Design review of the part built by this model. Coordinates are the model's own, in mm. A direction names the side the tool comes from. Coordinates: 2 decimals unless noted, no trailing zeros. Loops run counter-clockwise (first coordinate to the right, second up) from the corner with the lowest first, then second, coordinate; pieces in that order, holes last.
Q1. Add section C-C on z = -29.5. Give the boundary of the cut face in (x, y).
Q2. Wall thickness on probe 1 along X at (y, z) = (1.5, -139.7); probe 2 along X at (y, z) = (4.5, -114.3): over which ranges is each line inside the solid? List them lowest first.
Q3. For P1, Ø2.5, axis at x = -144, y = 5, coming from the -Z side; P2, Ø2, axis at y = 1, z = -86.5, coming from the -X side; P3, Ø3, axis at y = 4.5, z = -162.5, coming from the -X side; P4, Ø2.5, axis at y = 4.5, z = -20.5, coming from the +X side, all flat-tipped, find the tip position at first contact; note any pin that passes through.
Q4. Add section A-A on x = -139.7. Give the boundary of the cut face in (y, z), and give its area (3 significant figures).
Q5. Machinability: for faces 1 (the face through (-25.4, 4, -126)), 2 (the face through (-21, 4, -160)), 3 (the face through (-3, 4, -80)), which of the approach directions +Z, -Z, +X, -X, +Y, -Y give a long, thin tool a straight path to every point of the face, cutting with its end or side? Answer none if there is none.
Q6. Add section D-D on x = -29. Give the boundary of the cut face in (y, z).
Q7. Draft analysis for pull direction Z (two halves, no side actions). For faces 4 (the face through (0, 4, -50)), 5 (the face through (-24.285, 4.024, -105.16)), 6 (the face through (-1.804, 4.024, -1.711)), state which applies: released by +Z, released by -Z, zero draft, split by the parting line, or undercut.
Q8. Add section B-B on y = 2. Give the number of separate pieces and of enclosed holes in the cut face, and give its area (3 significant figures).
Autodesk Inventor part; units mm, degrees
ref_plane "YZ Plane" through (0, 0, 0) normal (1, 0, 0) x (0, 1, 0)
ref_plane "XZ Plane" through (0, 0, 0) normal (0, 1, 0) x (-1, 0, 0)
ref_plane "XY Plane" through (0, 0, 0) normal (0, 0, 1) x (1, 0, 0)
sketch "Sketch1" plane through (0, 0, 0) normal (0, 1, 0) x (-1, 0, 0)
  line L0 (169.8625, 0) -> (0, 0)
  line L1 (0, 0) -> (0, -169.8625)
  line L2 (0, -169.8625) -> (25.4, -169.8625)
  line L3 (25.4, -169.8625) -> (25.4, -103.8713)
  line L4 (103.8713, -25.4) -> (169.8625, -25.4)
  line L5 (169.8625, -25.4) -> (169.8625, 0)
  arc A0 (103.8713, -25.4) -> (25.4, -103.8713) centre (66.675, -66.675) ccw
  line L6 (0, 0) -> (66.675, -66.675) construction
  line L7 (0, -20) -> (6.35, -20)
  line L8 (6.35, -20) -> (6.35, -40)
  line L9 (6.35, -40) -> (0, -40)
  line L10 (0, -40) -> (0, -20)
  line L11 (6.35, -60) -> (6.35, -80)
  line L12 (0, -60) -> (6.35, -60)
  line L13 (6.35, -80) -> (0, -80)
  line L14 (6.35, -100) -> (6.35, -120)
  line L15 (0, -100) -> (6.35, -100)
  line L16 (6.35, -120) -> (0, -120)
  line L17 (6.35, -140) -> (6.35, -160)
  line L18 (0, -140) -> (6.35, -140)
  line L19 (6.35, -160) -> (0, -160)
  line L20 (23.368, -27.3469) -> (16.764, -27.3469)
  line L21 (16.764, -27.3469) -> (16.764, -12.0929)
  line L22 (16.764, -12.0929) -> (23.368, -12.0929)
  line L23 (23.368, -12.0929) -> (23.368, -27.3469)
  line L24 (23.368, -27.3469) -> (16.764, -12.0929) construction
  line L25 (16.764, -27.3469) -> (23.368, -12.0929) construction
  line L26 (25.4, -160) -> (16.764, -160)
  line L27 (16.764, -160) -> (16.764, -140)
  line L28 (16.764, -140) -> (25.4, -140)
  point P0 (103.8713, -25.4)
  point P1 (20.066, -19.7199)
  point P2 (20.066, -12.0929)
  dimension "d0" = 25.4
  dimension "d1" = 169.8625
  dimension "d2" = 25.4
  dimension "d3" = 169.8625
  dimension "d4" = 111.125
  dimension "d5" = 66.675
  dimension "d6" = 45
  dimension "d10" = 6.35
  dimension "d11" = 20
  dimension "d12" = 20
  dimension "d15" = 40
  dimension "d34" = 12.0929
  dimension "d35" = 6.604
  dimension "d36" = 20.066
  dimension "d37" = 15.254
extrude "Plate1" add sketch "Sketch1" along normal blind 7.9375 contours L5 L4 A0 L3 L28 L27 L26 L2 L1 L19 L17 L18 L16 L14 L15 L13 L11 L12 L9 L8 L7 L0
fillet "Corner Round1" radius 25.4 2 edges at (-103.8713, 3.9688, -25.4) (-25.4, 3.9688, -103.8713)
fillet "Corner Round2" radius 6 5 edges at (0, 3.9688, 0) (0, 3.9688, -169.8625) (-25.4, 3.9688, -169.8625) (-169.8625, 3.9688, 0) (-169.8625, 3.9688, -25.4)
sketch "Sketch2" plane through (0, 0, 0) normal (0, -1, 0) x (1, 0, 0)
  line L0 (-169.8625, -19.4) -> (-169.8625, -6)
  line L1 (-19.4, -169.8625) -> (-6, -169.8625)
  line L2 (-6, -169.8625) -> (-19.4, -169.8625)
  point P0 (0, 0)
  point P1 (-165.1, -12.7)
  point P2 (-139.7, -12.7)
  point P3 (-114.3, -12.7)
  point P4 (-12.7, -165.1)
  point P5 (-12.7, -139.7)
  point P6 (-12.7, -114.3)
  point P7 (-169.8625, -12.7)
  point P8 (-169.8625, -12.7)
  point P9 (-12.7, -169.8625)
  dimension "d21" = 25.4
  dimension "d22" = 25.4
  dimension "d23" = 25.4
  dimension "d24" = 25.4
  dimension "d25" = 4.7625
  dimension "d26" = 4.7625
hole "Hole1" at (-165.1, 0, -12.7) at (-139.7, 0, -12.7) at (-114.3, 0, -12.7) at (-12.7, 0, -165.1) at (-12.7, 0, -139.7) at (-12.7, 0, -114.3) direction (0, 1, 0) diameter 5.105 depth 7.9375 tip angle 118
equation "\"d2\" = d0"
equation "\"d3\" = d1"
equation "\"d12\" = d11"
equation "\"d15\" = 2 * d11"
equation "\"d32\" = Thickness"
equation "\"d8\" = Thickness"
equation "\"BendRadius\" = Thickness"
equation "\"BendReliefWidth\" = Thickness"
equation "\"BendReliefDepth\" = 0.5 * Thickness"
equation "\"CornerReliefSize\" = 4 * Thickness"
equation "\"MinimumRemnant\" = 2 * Thickness"
equation "\"TransitionRadius\" = BendRadius"
equation "\"JacobiRadiusSize\" = BendRadius"
equation "\"GapSize\" = Thickness"
properties part number "INTAKE_SWERVE_MOUNT" material "Aluminum, 6061-T6"
Entries:
1. outline: (-25.38, 0) - (-6.35, 0) - (-6.35, 7.94) - (-25.38, 7.94) - close
2. probe 1: x = -25.4 to -15.25, -10.15 to 0
2. probe 2: x = -25.4 to -15.25, -10.15 to -6.35
3. P1: stops at z = -25.4
3. P2: stops at x = -15.16
3. P3: stops at x = -25.4
3. P4: stops at x = 0
4. outline: (0, -25.4) - (7.94, -25.4) - (7.94, -15.25) - (0, -15.25) - close; (0, -10.15) - (7.94, -10.15) - (7.94, 0) - (0, 0) - close
4. area: 161 mm2
5. face 1: -Z, -X, +Y, -Y
5. face 2: -X, +Y, -Y
5. face 3: +X, +Y, -Y
6. outline: (0, -25.84) - (7.94, -25.84) - (7.94, 0) - (0, 0) - close
7. face 4: zero draft
7. face 5: undercut
7. face 6: released by +Z
8. separate pieces: 1
8. enclosed holes: 7
8. area: 5,580 mm2
